```python
from build123d import *

# Parameters (mm, degrees)
CROQUIS1_W              = 23
CROQUIS1_H              = 16
SALIENTE_EXTRUIR1_DEPTH = 15
CROQUIS2_W              = 11
CROQUIS2_H              = 12
CORTAR_EXTRUIR1_DEPTH   = 21
CROQUIS4_R              = 4
CORTAR_EXTRUIR2_DEPTH   = 23
CROQUIS5_W              = 5
CROQUIS5_H              = 12
CORTAR_EXTRUIR3_DEPTH   = 2
SALIENTE_EXTRUIR2_DEPTH = 15
CROQUIS7_W              = 2
CROQUIS7_H              = 16
SALIENTE_EXTRUIR3_DEPTH = 2


with BuildPart() as part:
    # Croquis1 → Saliente-Extruir1 (new body)
    with BuildSketch(Plane.XY):
        with Locations((11.5, 8)):
            Rectangle(CROQUIS1_W, CROQUIS1_H)
    extrude(amount=SALIENTE_EXTRUIR1_DEPTH)

    # Croquis2 → Cortar-Extruir1 (cut)
    with BuildSketch(Plane(origin=(23, 0, 0), x_dir=(0, 0, -1), z_dir=(1, 0, 0))):
        with Locations((-7.5, 8)):
            Rectangle(CROQUIS2_W, CROQUIS2_H)
    extrude(amount=-CORTAR_EXTRUIR1_DEPTH, mode=Mode.SUBTRACT)

    # Croquis4 → Cortar-Extruir2 (cut)
    with BuildSketch(Plane.ZY):
        with Locations((7.5, 8)):
            Circle(CROQUIS4_R)
    extrude(amount=-CORTAR_EXTRUIR2_DEPTH, mode=Mode.SUBTRACT)

    # Croquis5 → Cortar-Extruir3 (cut)
    with BuildSketch(Plane.XY.offset(15)):
        with Locations((20.5, 8)):
            Rectangle(CROQUIS5_W, CROQUIS5_H)
    extrude(amount=-CORTAR_EXTRUIR3_DEPTH, mode=Mode.SUBTRACT)

    # Croquis6 → Saliente-Extruir2 (add)
    with BuildSketch(Plane.XY.offset(15)):
        Polygon((20.184075088, 16), (20.184075088, 18), (27, 18), (27, 14), (25, 14), (25, 16), (23, 16), align=None)
        Polygon((20.184075088, 0), (23, 0), (25, 0), (25, 2), (27, 2), (27, -2), (20.184075088, -2), align=None)
    extrude(amount=-SALIENTE_EXTRUIR2_DEPTH)

    # Croquis7 → Saliente-Extruir3 (add)
    with BuildSketch(Plane(origin=(0, 0, 0), x_dir=(-1, 0, 0), z_dir=(0, 0, -1))):
        with Locations((-24, 8)):
            Rectangle(CROQUIS7_W, CROQUIS7_H)
    extrude(amount=-SALIENTE_EXTRUIR3_DEPTH)


solid = part.part
```
The listing builds one solid part. Answer for the finished solid, in the listing's coordinates (mm). A direction names the side the tool comes from. Give positions to 0.01 mm unless a question says otherwise; leave off trailing zeros. Loops run counter-clockwise (first coordinate to the right, second up) from the corner with the lowest first, then second, coordinate; pieces in that order, holes last. Notation, with made-up numbers: (29.5, 42.5) - (35.5, 42.5) arc R28 ccw to (35.5, 70.5) - close; hole circle Ø10 at (11, 24.25). An arc over 180 degrees is marked (long way). Return JSON: item names as keys, results as strings. Group by question number.
1. Find section C-C (x = 5.75). Write down the section's boundary in (y, z).
2. Find section D-D (y = 15.5). Write down the section's boundary in (x, z), then the cut area to 3 significant figures.
3. Find section A-A (y = 8). Write down the section's boundary in (x, z), then the cut area to 3 significant figures.
4. Straight lines are drawn through the part: line 1 (Y direction, x = 0.9, z = 7.5); line 2 (Y direction, x = 14.75, z = 5.75); line 3 (Z direction, x = 9.25, y = 8.75). For each, find the intervals that lie inside material, in ascending order. Write a range as [from, to].
5. Which of the six approach directions +Z, -Z, +X, -X, +Y, -Y give full straight-line access (tool end or side, diameter ignored) to faces 5 (the flat face through (24, 0, 9)), 6 (the flat face through (10, 0, 7)), 7 (the flat face through (26, 14, 8))?
6. Given pin 1 Ø1.6 at (y, z) = (5.5, 13.5) entering from +X; pin 2 Ø1.6 at (y, z) = (5.5, 1) entering from +X; pin 3 Ø5 at (x, z) = (17, 6.5) entering from +Y, each flat-ended and moving along its own axis, determine where each tip first touches the part or whether it passes through.
7. Find section B-B (z = 7.5). Write down the section's boundary in (x, y).
8. Determine the mould class of faces 1 (the flat face through (24, 16, 9)), 2 (the flat face through (25, 8, 1)), 3 (the flat face through (11, 8, 15)), 4 (the flat face through (20.184, 17, 8)) for opening direction X: pulls with the +X half, pulls with the -X half, needs draft (parallel to the pull), parting line crosses it, or undercut.
Verdict:
{
 "1": {"outline": "(0, 0) - (16, 0) - (16, 15) - (0, 15) - close; hole (2, 2) - (14, 2) - (14, 13) - (2, 13) - close"},
 "2": {"outline": "(0, 0) - (27, 0) - (27, 15) - (25, 15) - (25, 2) - (23, 2) - (23, 15) - (0, 15) - close", "area": "379 mm^2"},
 "3": {"outline": "(0, 0) - (25, 0) - (25, 2) - (2, 2) - (2, 3.5) - (0, 3.5) - close; (0, 11.5) - (2, 11.5) - (2, 13) - (18, 13) - (18, 15) - (0, 15) - close", "area": "92.0 mm^2"},
 "4": {"line 1": "y = [0, 4], [12, 16]", "line 2": "y = [0, 2], [14, 16]", "line 3": "z = [0, 2], [13, 15]"},
 "5": {"face 5": "+Z", "face 6": "+Z, -Z, -X, -Y", "face 7": "+Z, -Z, +X"},
 "6": {"pin 1": "stops at x = 18", "pin 2": "stops at x = 25", "pin 3": "stops at y = 16"},
 "7": {"outline": "(0, 0) - (20.18, 0) - (20.18, -2) - (27, -2) - (27, 2) - (25, 2) - (25, 0) - (23, 0) - (23, 2) - (2, 2) - (2, 4) - (0, 4) - close; (0, 12) - (2, 12) - (2, 14) - (23, 14) - (23, 16) - (25, 16) - (25, 14) - (27, 14) - (27, 18) - (20.18, 18) - (20.18, 16) - (0, 16) - close"},
 "8": {"face 1": "undercut", "face 2": "pulls with the +X half", "face 3": "needs draft", "face 4": "pulls with the -X half"}
}
